```python
from build123d import *

# Parameters (mm, degrees)
F0_W     = 5
F0_H     = 4.0733553469
F0_W_2   = 6.2
F0_H_2   = 13
F1_DEPTH = 25
F2_DEPTH = 8
F3_R     = 1


with BuildPart() as f1:
    # F0 (on Front) → F1 (new body)
    with BuildSketch(Plane.XZ):
        with Locations((-13.7, -2.0366776735)):
            Rectangle(F0_W, F0_H)
        Polygon((38.7, 15.7062858343), (-11.2, 15.7062858343), (-11.2, 0), (-11.2, -4.0733553469), (38.7, -4.0733553469), (38.7, 0), align=None)
        Polygon((27.5, 0), (0, 0), (-6.2, 0), (-6.2, 13), (0, 13), (27.5, 13), (33.7, 13), (33.7, 0), align=None, mode=Mode.SUBTRACT)
        with Locations((41.2, -2.0366776735)):
            Rectangle(F0_W, F0_H)
        with Locations((-3.1, 6.5)):
            Rectangle(F0_W_2, F0_H_2)
        with Locations((30.6, 6.5)):
            Rectangle(F0_W_2, F0_H_2)
    extrude(amount=F1_DEPTH)

    # F0 (on Front) → F2 (cut)
    with BuildSketch(Plane.XZ):
        with Locations((30.6, 6.5)):
            Rectangle(F0_W_2, F0_H_2)
        with Locations((-3.1, 6.5)):
            Rectangle(F0_W_2, F0_H_2)
    extrude(amount=F2_DEPTH, mode=Mode.SUBTRACT)

    # F3
    f3_edges = [f1.edges().sort_by_distance(p)[0] for p in [
        (38.7, -12.5, 15.706286),
        (-11.2, -12.5, 15.706286),
        (13.75, 0, 15.706286),
        (13.75, -25, 15.706286),
        (38.7, -12.5, 0),
        (38.7, 0, 7.853143),
        (38.7, -25, 7.853143),
        (43.7, -12.5, 0),
        (41.2, 0, 0),
        (41.2, -25, 0),
        (43.7, -12.5, -4.073355),
        (43.7, 0, -2.036678),
        (43.7, -25, -2.036678),
        (-11.2, -12.5, 0),
        (-11.2, 0, 7.853143),
        (-11.2, -25, 7.853143),
        (-16.2, -12.5, 0),
        (-16.2, -12.5, -4.073355),
        (-16.2, 0, -2.036678),
        (-16.2, -25, -2.036678),
        (-13.7, 0, 0),
        (-13.7, -25, 0),
    ]]
    fillet(f3_edges, radius=F3_R)


solid = f1.part
```
Geometry: final body of the model. Coordinates: model frame, mm. A direction names the side the tool comes from. Coordinates: 2 decimals unless noted, no trailing zeros. Write each loop counter-clockwise with the first axis right and the second up, starting at its lowest first coordinate (ties: lowest second). Pieces come first, ordered by that corner, then holes. Notation, with made-up numbers: M 8.25,-5.5 L 22.25,-5.5 A26 cw 22.25,30.5 Z; hole C 51,48 d1. An arc over 180 degrees is marked long. Use CSV: the item, a comma, the result in double quotes. Start each with the question number.
1. Ray query, probe 1 along X at (y, z) = (-20, 10); probe 2 along Z at (x, y) = (33.5, -1.5); probe 3 along X at (y, z) = (-1.5, 2.5). Return the intervals inside material, ascending.
2. Cut plane C-C on x = 7.5. Return the cut outline in (y, z), plus the area to 3 significant figures.
3. Cut plane D-D on z = 14. Return the cut outline in (x, y).
4. First-contact query: P1, Ø3, axis at y = -21.5, z = 13.5, coming from the +X side; P2, Ø4, axis at y = -21, z = 13.5, coming from the -X side; P3, Ø2.5, axis at x = -13, y = -8.5, coming from the +Z side. Flat tips, straight axial feed; report the tip coordinate or a pass-through.
5. Cut plane B-B on y = -5.25. Return the cut outline in (x, z), plus the area to 3 significant figures.
6. Reachability of faces 1 (the face through (-11.2, -12, 8)), 2 (the face through (-3, -8, 7)), 3 (the face through (27.5, -16, 6)) from +Z, -Z, +X, -X, +Y, -Y: full face, straight path, thin tool, end or side. Return the list, or none.
7. Mould query, pull axis Z, two halves, no side actions, for faces 4 (the face through (-14, -12, 0)), 5 (the face through (13, -12, -4.073)), 6 (the face through (13, -12, 0)), 7 (the face through (31, -8, 7)). Classes: pulls with the +Z half, pulls with the -Z half, needs draft (parallel to the pull), parting line crosses it, or undercut.
8. Cut plane A-A on z = 3. Return the cut outline in (x, y).
Entries:
1,probe 1,"-11.2 to 0, 27.5 to 38.7"
1,probe 2,"-4.07 to 0, 13 to 15.71"
1,probe 3,"-11.2 to -6.2, 33.7 to 38.7"
2,outline,"M -25,-4.07 L 0,-4.07 L 0,0 L -25,0 Z; M -25,13 L 0,13 L 0,14.71 A1 ccw -1,15.71 L -24,15.71 A1 ccw -25,14.71 Z"
2,area,"169 mm²"
3,outline,"M -11.2,-24 A1 ccw -10.2,-25 L 37.7,-25 A1 ccw 38.7,-24 L 38.7,-1 A1 ccw 37.7,0 L -10.2,0 A1 ccw -11.2,-1 Z"
4,P1,"x = 38.7"
4,P2,"x = -11.2"
4,P3,"z = 0.11"
5,outline,"M -16.2,-3.07 A1 ccw -15.2,-4.07 L 42.7,-4.07 A1 ccw 43.7,-3.07 L 43.7,-1 A1 ccw 42.7,0 L 39.7,0 A1 cw 38.7,1 L 38.7,14.71 A1 ccw 37.7,15.71 L -10.2,15.71 A1 ccw -11.2,14.71 L -11.2,1 A1 cw -12.2,0 L -15.2,0 A1 ccw -16.2,-1 Z; hole M -6.2,0 L 33.7,0 L 33.7,13 L -6.2,13 Z"
5,area,"508 mm²"
6,face 1,"+Z, -X, +Y, -Y"
6,face 2,"+Y"
6,face 3,"+Y, -Y"
7,face 4,"pulls with the +Z half"
7,face 5,"pulls with the -Z half"
7,face 6,"undercut"
7,face 7,"undercut"
8,outline,"M -11.2,-24 A1 ccw -10.2,-25 L 0,-25 L 0,-8 L -6.2,-8 L -6.2,0 L -10.2,0 A1 ccw -11.2,-1 Z; M 27.5,-25 L 37.7,-25 A1 ccw 38.7,-24 L 38.7,-1 A1 ccw 37.7,0 L 33.7,0 L 33.7,-8 L 27.5,-8 Z"
